from build123d import *

# Parameters (mm, degrees)
CROQUIS1_R              = 25
SALIENTE_EXTRUIR1_DEPTH = 3
CROQUIS2_W              = 12.95
CROQUIS2_H              = 12.95
SALIENTE_EXTRUIR2_DEPTH = 3
CROQUIS3_R              = 1.5
CROQUIS3_R_2            = 2
CORTAR_EXTRUIR1_DEPTH   = 124.455998815


with BuildPart() as part:
    # Croquis1 → Saliente-Extruir1 (new body)
    with BuildSketch(Plane.XY):
        with BuildLine():
            Line((-15.070986718, 74.306476298), (-15.070986718, 37.256476298))
            ThreePointArc((-15.070986718, 37.256476298), (-28.445175059, 28.391049341), (-37.285113206, 15))
            Line((-37.285113206, 15), (-74.335113206, 15))
            Line((-74.335113206, 15), (-74.335113206, 20.59))
            Line((-74.335113206, 20.59), (-87.285113206, 20.59))
            Line((-87.285113206, 20.59), (-87.285113206, -20.59))
            Line((-87.285113206, -20.59), (-74.335113206, -20.59))
            Line((-74.335113206, -20.59), (-74.335113206, -15))
            Line((-74.335113206, -15), (-37.285113206, -15))
            ThreePointArc((-37.285113206, -15), (-28.445175059, -28.391049341), (-15.070986718, -37.256476298))
            Line((-15.070986718, -37.256476298), (-15.070986718, -74.306476298))
            Line((-15.070986718, -74.306476298), (-20.660986718, -74.306476298))
            Line((-20.660986718, -74.306476298), (-20.660986718, -87.256476298))
            Line((-20.660986718, -87.256476298), (20.519013282, -87.256476298))
            Line((20.519013282, -87.256476298), (20.519013282, -74.306476298))
            Line((20.519013282, -74.306476298), (14.929013282, -74.306476298))
            Line((14.929013282, -74.306476298), (14.929013282, -37.256476298))
            ThreePointArc((14.929013282, -37.256476298), (28.353570497, -28.407666286), (37.22795272, -15))
            Line((37.22795272, -15), (59.27795272, -15))
            Line((59.27795272, -15), (59.27795272, -20.59))
            Line((59.27795272, -20.59), (72.22795272, -20.59))
            Line((72.22795272, -20.59), (72.22795272, 20.59))
            Line((72.22795272, 20.59), (59.27795272, 20.59))
            Line((59.27795272, 20.59), (59.27795272, 15))
            Line((59.27795272, 15), (37.22795272, 15))
            ThreePointArc((37.22795272, 15), (28.353570497, 28.407666286), (14.929013282, 37.256476298))
            Line((14.929013282, 37.256476298), (14.929013282, 74.306476298))
            Line((14.929013282, 74.306476298), (20.519013282, 74.306476298))
            Line((20.519013282, 74.306476298), (20.519013282, 87.256476298))
            Line((20.519013282, 87.256476298), (-20.660986718, 87.256476298))
            Line((-20.660986718, 87.256476298), (-20.660986718, 74.306476298))
            Line((-20.660986718, 74.306476298), (-15.070986718, 74.306476298))
        make_face()
        Circle(CROQUIS1_R, mode=Mode.SUBTRACT)
    extrude(amount=SALIENTE_EXTRUIR1_DEPTH)

    # Croquis2 → Saliente-Extruir2 (add)
    with BuildSketch(Plane(origin=(0, 0, 0), x_dir=(-1, 0, 0), z_dir=(0, 0, -1))):
        with Locations((-26.994013282, 80.781476298)):
            Rectangle(CROQUIS2_W, CROQUIS2_H)
        with Locations((27.135986718, 80.781476298)):
            Rectangle(CROQUIS2_W, CROQUIS2_H)
        with Locations((-26.994013282, -80.781476298)):
            Rectangle(CROQUIS2_W, CROQUIS2_H)
        with Locations((27.135986718, -80.781476298)):
            Rectangle(CROQUIS2_W, CROQUIS2_H)
        with Locations((80.810113206, 27.065)):
            Rectangle(CROQUIS2_W, CROQUIS2_H)
        with Locations((80.810113206, -27.065)):
            Rectangle(CROQUIS2_W, CROQUIS2_H)
    extrude(amount=-SALIENTE_EXTRUIR2_DEPTH)

    # Croquis3 → Cortar-Extruir1 (cut, through all)
    with BuildSketch(Plane(origin=(0, 0, 0), x_dir=(-1, 0, 0), z_dir=(0, 0, -1))):
        with Locations((-26.994013282, 80.781476298)):
            Circle(CROQUIS3_R)
        with Locations((27.135986718, 80.781476298)):
            Circle(CROQUIS3_R_2)
        with Locations((27.135986718, -80.781476298)):
            Circle(CROQUIS3_R_2)
        with Locations((-26.994013282, -80.781476298)):
            Circle(CROQUIS3_R_2)
        with Locations((80.810113206, -27.065)):
            Circle(CROQUIS3_R_2)
        with Locations((80.810113206, 27.065)):
            Circle(CROQUIS3_R_2)
    extrude(amount=-CORTAR_EXTRUIR1_DEPTH, mode=Mode.SUBTRACT)


solid = part.part
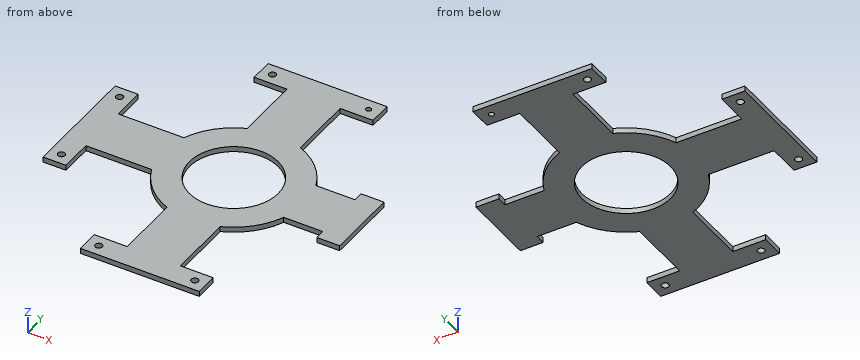
Could you check a few things on this model? Use its own coordinates, in mm. Round coordinates to 2 decimals unless told otherwise and drop trailing zeros. Loops run counter-clockwise (first coordinate to the right, second up) from the corner with the lowest first, then second, coordinate; pieces in that order, holes last. Notation, with made-up numbers: (3.25, 1.5) -> (13.25, 1.5) arc R20 cw to (13.25, 28.5) -> close; hole circle Ø9 at (57.5, 68.5). An arc over 180 degrees is marked (long way). Use CSV: the item, a comma, the result in double quotes.
(1) Suppose I cut it at C-C on x = 21.5. Write out the boundary of the cut face in (y, z).
Return value:
outline,"(-87.26, 0) -> (-74.31, 0) -> (-74.31, 3) -> (-87.26, 3) -> close; (-33.89, 0) -> (-12.76, 0) -> (-12.76, 3) -> (-33.89, 3) -> close; (12.76, 0) -> (33.89, 0) -> (33.89, 3) -> (12.76, 3) -> close; (74.31, 0) -> (87.26, 0) -> (87.26, 3) -> (74.31, 3) -> close"
(2) Suppose I cut it at D-D on z = 0.95. Give the number of separate pieces and of enclosed holes in the cut face, plus the area to 3 significant figures.
Return value:
separate pieces,"1"
enclosed holes,"7"
area,"9,940 mm²"
(3) Suppose I cut it at A-A on y = 0. Write out the boundary of the cut face in (x, z).
Return value:
outline,"(-87.29, 0) -> (-25, 0) -> (-25, 3) -> (-87.29, 3) -> close; (25, 0) -> (72.23, 0) -> (72.23, 3) -> (25, 3) -> close"
(4) Suppose I cut it at B-B on x = 0. Write out the boundary of the cut face in (y, z), plus the area to 3 significant figures.
Return value:
outline,"(-87.26, 0) -> (-25, 0) -> (-25, 3) -> (-87.26, 3) -> close; (25, 0) -> (87.26, 0) -> (87.26, 3) -> (25, 3) -> close"
area,"374 mm²"
(5) Will these pins go through, and if not, where does the flat tip stop? pin 1 Ø0.9 at (x, z) = (-78.5, 1.5) entering from +Y; pin 2 Ø0.9 at (y, z) = (56.5, 1.5) entering from -X; pin 3 Ø0.9 at (y, z) = (-80.5, 1.5) entering from -X; pin 4 Ø1.5 at (x, y) = (37.5, -16.5) entering from +Z (3 decimals).
Return value:
pin 1,"stops at y = 33.54"
pin 2,"stops at x = -15.07"
pin 3,"stops at x = -33.61"
pin 4,"passes through"
(6) If I drill on probe 1 along Y at (x, z) = (0, 1.2); probe 2 along Y at (x, z) = (-32, 2.4); probe 3 along X at (y, z) = (-69, 1.7), over which ranges is the centre line in solid material (lowest first)? Write a range as [from, to].
Return value:
probe 1,"y = [-87.26, -25], [25, 87.26]"
probe 2,"y = [-87.26, -74.31], [-24.31, 24.31], [74.31, 87.26]"
probe 3,"x = [-15.07, 14.93]"
